The drawing under review shows one solid part. Ordinate dimensions are in mm from its lowest x, y, z. Round coordinates to 2 decimals unless told otherwise and drop trailing zeros. Order: outer loops, then holes, each group sorted by start corner. A loop starts at its lowest first (then second) coordinate and runs counter-clockwise, first axis right, second up. Notation, with made-up numbers: M -24.75,13.5 L 1.25,13.5 A25 ccw 1.25,26.5 Z; hole C -14.75,0 d8. An arc over 180 degrees is marked long. Write item = value, one per line. Start each with the question number.
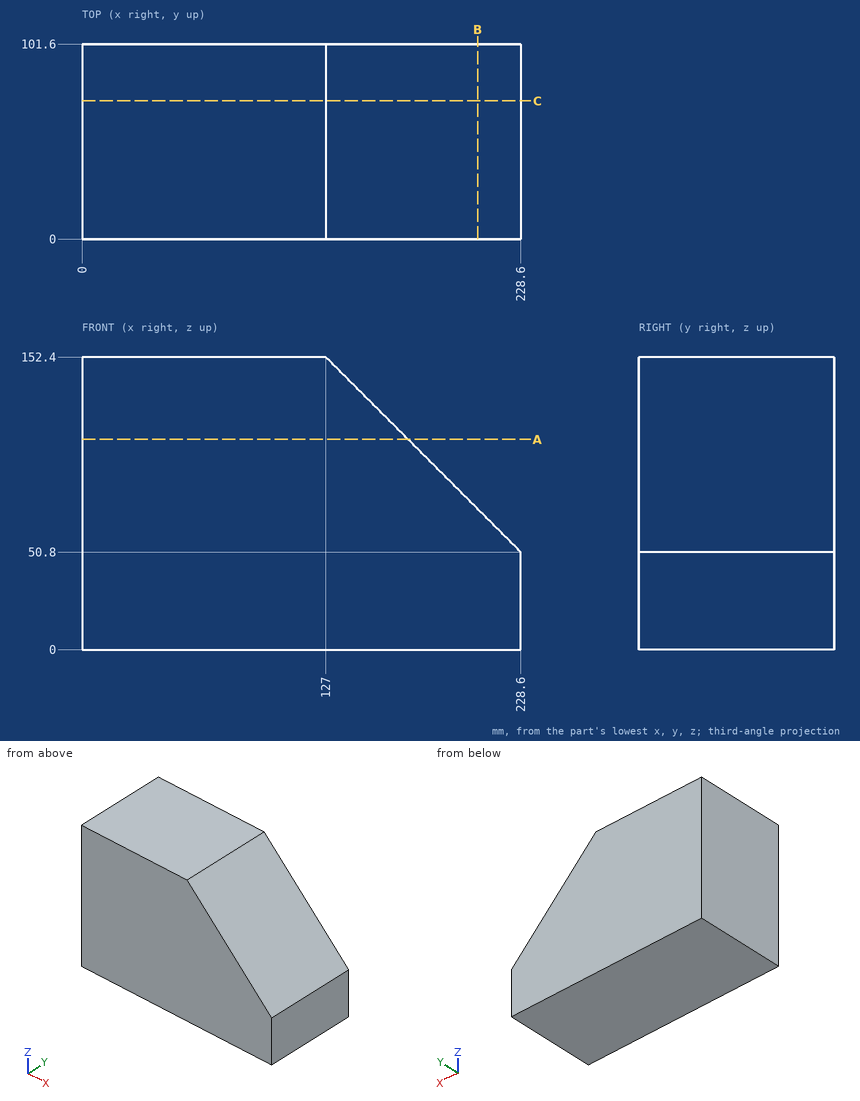
(1) For line 1 along X through (y, z) = (64.5, 78.5); line 2 along X through (y, z) = (90, 117.5); line 3 along Z through (x, y) = (167.5, 46.5), list the stretches that pass through material, from the lowest coordinate up. Write a range as [from, to].
(2) Insertion check: pin 1 (8 mm diameter, centred on y = 77, z = 103.5, fed in from +X); pin 2 (1 mm diameter, centred on x = 157.5, y = 26.5, fed in from +Z). Each pin has a flat end and moves straight along its axis. Give the tip position at first contact, or say it passes through.
(3) Consider section C-C, the plane y = 72. Write out the cut boundary in (x, z), then the cut area to 3 significant figures.
(4) Consider section B-B, the plane x = 206. Write out the cut boundary in (y, z).
(5) Consider section A-A, the plane z = 109.5. Write out the cut boundary in (x, y), then the cut area to 3 significant figures.
Completed:
q1.line_1 = [0, 200.9]
q1.line_2 = [0, 161.9]
q1.line_3 = [0, 111.9]
q2.pin_1 = 179.9
q2.pin_2 = 122.4
q3.outline = M 0,0 L 228.6,0 L 228.6,50.8 L 127,152.4 L 0,152.4 Z
q3.area = 29,700 mm2
q4.outline = M 0,0 L 101.6,0 L 101.6,73.4 L 0,73.4 Z
q5.outline = M 0,0 L 169.9,0 L 169.9,101.6 L 0,101.6 Z
q5.area = 17,300 mm2
